```python
from build123d import *

# Parameters (mm, degrees)
SKETCH_R     = 1.1
PAD_DEPTH    = 6
POCKET_DEPTH = 5
FILLET_R     = 1


with BuildPart() as part:
    # Sketch → Pad (new body)
    with BuildSketch(Plane.XY):
        with BuildLine():
            ThreePointArc((4.5, 10.5), (0, 15), (-4.5, 10.5))
            Line((-4.5, 10.5), (-4.5, -10.5))
            ThreePointArc((-4.5, -10.5), (0, -15), (4.5, -10.5))
            Line((4.5, -10.5), (4.5, 10.5))
        make_face()
        with Locations((0, 10.5)):
            Circle(SKETCH_R, mode=Mode.SUBTRACT)
        with Locations((0, -10.5)):
            Circle(SKETCH_R, mode=Mode.SUBTRACT)
    extrude(amount=PAD_DEPTH)

    # Sketch001 (on Face8 of Pad) → Pocket (cut)
    with BuildSketch(Plane.XY.offset(6)):
        with BuildLine():
            ThreePointArc((3.5, 10.5), (0, 14), (-3.5, 10.5))
            Line((-3.5, 10.5), (-2, -3))
            ThreePointArc((-2, -3), (0, -5), (2, -3))
            Line((3.5, 10.5), (2, -3))
        make_face()
    extrude(amount=-POCKET_DEPTH, mode=Mode.SUBTRACT)

    # Fillet
    fillet_edges = [part.edges().sort_by_distance(p)[0] for p in [
        (4.5, 0, 0),
    ]]
    fillet(fillet_edges, radius=FILLET_R)


solid = part.part
```
Here's how the part is built. I have some questions about the finished solid (model axes, mm). A direction names the side the tool comes from. Round coordinates to 2 decimals unless told otherwise and drop trailing zeros. Write each loop counter-clockwise with the first axis right and the second up, starting at its lowest first coordinate (ties: lowest second). Pieces come first, ordered by that corner, then holes.
Q1. If we section it at B-B on z = 0.4: Write out the boundary of the cut face in (x, y).
Q2. If we section it at A-A on x = 0: Write out the boundary of the cut face in (y, z).
Q3. If we mould it in two halves opening along Y, with no side actions, what happens to faces 1 (the cylindrical face through (0, 14, 4)), 2 (the flat face through (4.5, 0, 3)), 3 (the cylindrical face through (0, -15, 3))? For each: +Y half, -Y half, draft (parallel to the pull), parting line (faces both ways), or undercut.
Q4. If we section it at C-C on y = 4.75: Write out the boundary of the cut face in (x, z).
Q5. Which directions (+Z, -Z, +X, -X, +Y, -Y) give clear straight access to the entire face, cutting with the end or side of a thin tool? Please do faces 4 (the cylindrical face through (-4.215, -0.147, 0.301)), 5 (the flat face through (0, 5, 1)).
Q6. Please list where these lines run through material, in increasing order: probe 1 along Y at (x, z) = (0, 1.8); probe 2 along Y at (x, z) = (0, 0.7); probe 3 along X at (y, z) = (-9.5, 1).
Q7. Will these pins go through, and if not, where does the flat tip stop? P1, Ø3.5, axis at x = 0, y = 10.5, coming from the -Z side; P2, Ø1, axis at x = 2.5, z = 5.5, coming from the +Y side; P3, Ø2, axis at x = -0.5, y = 2.5, coming from the +Z side.
Answer below:
1. outline: (-4.3, -10.5) arc R4.3 ccw to (4.3, -10.5) - (4.3, 10.5) arc R4.3 ccw to (-4.3, 10.5) - close; hole circle Ø2.2 at (0, -10.5); hole circle Ø2.2 at (0, 10.5)
2. outline: (-15, 1) arc R1 ccw to (-14, 0) - (-11.6, 0) - (-11.6, 6) - (-15, 6) - close; (-9.4, 0) - (9.4, 0) - (9.4, 1) - (-5, 1) - (-5, 6) - (-9.4, 6) - close; (11.6, 0) - (14, 0) arc R1 ccw to (15, 1) - (15, 6) - (14, 6) - (14, 1) - (11.6, 1) - close
3. face 1: undercut
3. face 2: draft
3. face 3: -Y half
4. outline: (-4.5, 1) arc R1 ccw to (-3.5, 0) - (3.5, 0) arc R1 ccw to (4.5, 1) - (4.5, 6) - (2.86, 6) - (2.86, 1) - (-2.86, 1) - (-2.86, 6) - (-4.5, 6) - close
5. face 4: -Z, -X, +Y, -Y
5. face 5: +Z
6. probe 1: y = -15 to -11.6, -9.4 to -5, 14 to 15
6. probe 2: y = -14.95 to -11.6, -9.4 to 9.4, 11.6 to 14.95
6. probe 3: x = -4.5 to -0.46, 0.46 to 4.5
7. P1: stops at z = 0
7. P2: stops at y = 14.53
7. P3: stops at z = 1
